The listing builds one solid part. Answer for the finished solid, in the listing's coordinates (mm). Give positions to 0.01 mm unless a question says otherwise; leave off trailing zeros. Write each loop counter-clockwise with the first axis right and the second up, starting at its lowest first coordinate (ties: lowest second). Pieces come first, ordered by that corner, then holes. Notation, with made-up numbers: (77, 23) - (134, 23) arc R29 ccw to (134, 44) - close; hole circle Ø8 at (34, -9.75). An arc over 180 degrees is marked (long way). Use a Markdown table: item, result. Add a question column.
from build123d import *

# Parameters (mm, degrees)
F0_R  = 14.2031372516
F5_R  = 5.7900940223
F6_R  = 5.811478977
F7_R  = 13.5706885585
F8_R  = 20.0607447558
F14_R = 25.3778243108
F16_R = 5


with BuildPart() as f9:
    # F0 (on Top) → F9 section 0
    with BuildSketch(Plane.XY):
        Circle(F0_R)
    # F5 (on offset) → F9 section 1
    with BuildSketch(Plane.XY.offset(-10)):
        Circle(F5_R)
    loft()

    # F5 (on offset) → F10 section 0
    with BuildSketch(Plane.XY.offset(-10)):
        Circle(F5_R)
    # F6 (on offset) → F10 section 1
    with BuildSketch(Plane.XY.offset(-110)):
        Circle(F6_R)
    loft()

    # F6 (on offset) → F11 section 0
    with BuildSketch(Plane.XY.offset(-110)):
        Circle(F6_R)
    # F7 (on offset) → F11 section 1
    with BuildSketch(Plane.XY.offset(-120)):
        Circle(F7_R)
    loft()

    # F7 (on offset) → F12 section 0
    with BuildSketch(Plane.XY.offset(-120)):
        Circle(F7_R)
    # F8 (on offset) → F12 section 1
    with BuildSketch(Plane.XY.offset(-220)):
        Circle(F8_R)
    loft()

    # F8 (on offset) → F15 section 0
    with BuildSketch(Plane.XY.offset(-220)):
        Circle(F8_R)
    # F14 (on offset) → F15 section 1
    with BuildSketch(Plane.XY.offset(-300)):
        Circle(F14_R)
    loft()

    # F16
    f16_edges = [f9.edges().sort_by_distance(p)[0] for p in [
        (-25.377824, 0, -300),
    ]]
    fillet(f16_edges, radius=F16_R)


solid = f9.part
1. For a pull along Z with two mould halves and no side action, classify faces 1 (the flat face through (0, 0, 0)), 2 (the flat face through (0, 0, -300)), 3 (the conical face through (-6.291, 0.277, -110.626)) as released by +Z, released by -Z, zero draft, split by the parting line, or undercut.
2. Given P1, Ø12, axis at x = 19.5, z = -234.5, coming from the +Y side; P2, Ø5, axis at y = 2.5, z = -205.5, coming from the -X side; P3, Ø8, axis at y = 19.5, z = -263, coming from the -X side, each flat-ended and moving along its own axis, determine where each tip first touches the part or whether it passes through.
3. The part is cut by section B-B (z = -216). Give the vertices of the cut face in (x, y), and give its area (3 significant figures).
4. The part is cut by section A-A (z = -145.5). Give the vertices of the cut face in (x, y).
5. Consider L1, parallel to Z at x = 1.5, y = -9; L2, parallel to X at y = 3.5, z = -137; L3, parallel to Y at x = 0.5, z = -19.5. Determine where each line is inside the solid, lowest interval first. Write a range as [from, to].
Check values:
| question | item | result |
|---|---|---|
| 1 | face 1 | released by +Z |
| 1 | face 2 | released by -Z |
| 1 | face 3 | undercut |
| 2 | P1 | stops at y = 16.14 |
| 2 | P2 | stops at x = -19.22 |
| 2 | P3 | stops at x = -16.9 |
| 3 | outline | circle Ø39.6 at (0, 0) |
| 3 | area | 1,230 mm2 |
| 4 | outline | circle Ø30.45 at (0, 0) |
| 5 | L1 | z = [-300, -114.27], [-6.04, 0] |
| 5 | L2 | x = [-14.25, 14.25] |
| 5 | L3 | y = [-5.77, 5.77] |
